```python
from build123d import *

# Parameters (mm, degrees)
SKETCH1_W                 = 57.404
SKETCH1_H                 = 90
BOSS_EXTRUDE1_DEPTH       = 1.5875
SKETCH2_W                 = 90
SKETCH2_H                 = 13.9065
BOSS_EXTRUDE2_DEPTH       = 1.5875
SKETCH3_W                 = 1.5875
SKETCH3_H                 = 13.9065
BOSS_EXTRUDE3_DEPTH       = 54.229
SKETCH4_W                 = 90
SKETCH4_H                 = 15.494
BOSS_EXTRUDE4_DEPTH       = 1.5875
F_8_CLEARANCE_HOLE1_D     = 4.4958
F_8_CLEARANCE_HOLE1_DEPTH = 1.5875


with BuildPart() as part:
    # Sketch1 → Boss-Extrude1 (new body)
    with BuildSketch(Plane(origin=(0, 0, 0), x_dir=(1, 0, 0), z_dir=(0, 1, 0))):
        with Locations((28.702, -45)):
            Rectangle(SKETCH1_W, SKETCH1_H)
    extrude(amount=BOSS_EXTRUDE1_DEPTH)

    # Sketch2 → Boss-Extrude2 (add)
    with BuildSketch(Plane(origin=(57.404, 0, 0), x_dir=(0, 0, -1), z_dir=(1, 0, 0))):
        with Locations((-45, 8.54075)):
            Rectangle(SKETCH2_W, SKETCH2_H)
    extrude(amount=-BOSS_EXTRUDE2_DEPTH)

    # Sketch3 → Boss-Extrude3 (add)
    with BuildSketch(Plane.ZY.offset(-55.8165)):
        with Locations((0.79375, 8.54075)):
            Rectangle(SKETCH3_W, SKETCH3_H)
        with Locations((89.20625, 8.54075)):
            Rectangle(SKETCH3_W, SKETCH3_H)
    extrude(amount=BOSS_EXTRUDE3_DEPTH)

    # Sketch4 → Boss-Extrude4 (add)
    with BuildSketch(Plane.ZY.offset(-1.5875)):
        with Locations((45, 7.747)):
            Rectangle(SKETCH4_W, SKETCH4_H)
    extrude(amount=BOSS_EXTRUDE4_DEPTH)

    # #8 Clearance Hole1
    with Locations(Plane(origin=(0, 1.5875, 0), x_dir=(1, 0, 0), z_dir=(0, 1, 0))):
        with Locations((28.702, -73.5203), (28.702, -15.875)):
            Hole(F_8_CLEARANCE_HOLE1_D / 2, depth=F_8_CLEARANCE_HOLE1_DEPTH)


solid = part.part
```
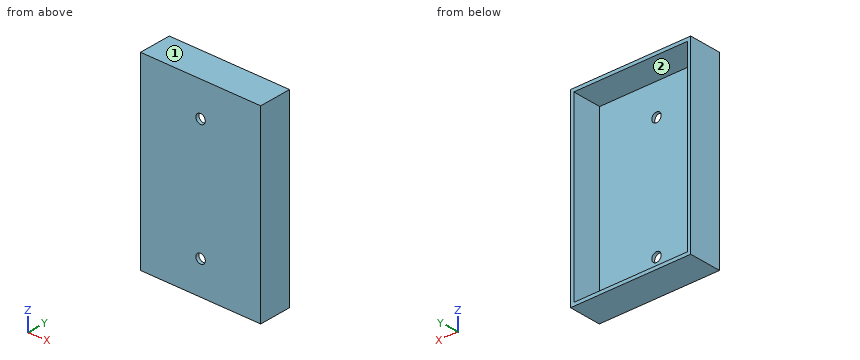
Geometry check sheet. Reference: the model listing, model coordinates, mm. Face numbers are marked on the shaded views. A direction names the side the tool comes from. Round coordinates to 2 decimals unless told otherwise and drop trailing zeros. Order: outer loops, then holes, each group sorted by start corner. A loop starts at its lowest first (then second) coordinate and runs counter-clockwise, first axis right, second up. Notation, with made-up numbers: M 26.5,83 L 57.5,83 A19 ccw 57.5,105 Z; hole C 87,41.25 d10. An arc over 180 degrees is marked long. Write item = value, one per line.
Q1. Section check A-A (y = 2.75). Enter the section's corners in (x, z), plus the area to 3 significant figures.
Answer block:
outline = M 0,0 L 57.4,0 L 57.4,90 L 0,90 Z; hole M 1.59,1.59 L 55.82,1.59 L 55.82,88.41 L 1.59,88.41 Z
area = 458 mm^2
Q2. Section check B-B (x = 41). Enter the section's corners in (y, z).
Answer block:
outline = M 0,0 L 15.49,0 L 15.49,1.59 L 1.59,1.59 L 1.59,88.41 L 15.49,88.41 L 15.49,90 L 0,90 Z
Q3. Depth check by flat-ended pin: pin 1 Ø2 at (x, y) = (48, 9) entering from -Z; pin 2 Ø1.5 at (x, z) = (50, 42) entering from +Y; pin 3 Ø4 at (x, z) = (28.702, 15.875) entering from -Y. Enter the tip coordinate at first touch or a pass-through.
Answer block:
pin_1 = 0
pin_2 = 1.59
pin_3 = through
Q4. Scan lines: line 1 (X direction, y = 9.75, z = 83.5); line 2 (Z direction, x = 7.5, y = 11); line 3 (Y direction, x = 49, z = 72.5). Record each from-to range of solid material in increasing order.
Answer block:
line_1 = 0 to 1.59, 55.82 to 57.4
line_2 = 0 to 1.59, 88.41 to 90
line_3 = 0 to 1.59
Q5. Set-up check for the marked faces 1 and 2: record each of +Z, -Z, +X, -X, +Y, -Y from which the full face is reachable in a straight line by a thin tool's end or side.
Answer block:
face_1 = +Z, +X, -X, +Y, -Y
face_2 = +Y
Q6. Section check C-C (z = 51.5). Enter the section's corners in (x, y).
Answer block:
outline = M 0,0 L 57.4,0 L 57.4,15.49 L 55.82,15.49 L 55.82,1.59 L 1.59,1.59 L 1.59,15.49 L 0,15.49 Z
